Read the model definition and answer for the solid it produces. Units are mm, in the model's axes. Face numbers are marked on the shaded views. A direction names the side the tool comes from. Coordinates: 2 decimals unless noted, no trailing zeros. Write each loop counter-clockwise with the first axis right and the second up, starting at its lowest first coordinate (ties: lowest second). Pieces come first, ordered by that corner, then holes. Notation, with made-up numbers: (42, 62.5) -> (91, 62.5) arc R13 cw to (91, 73.5) -> close; hole circle Ø2 at (42.5, 57.5). An arc over 180 degrees is marked (long way). Return JSON: item names as keys, results as strings.
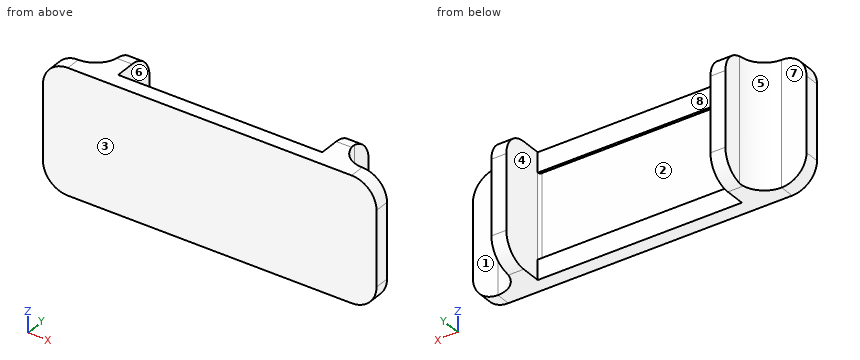
from build123d import *

# Parameters (mm, degrees)
BOSS_EXTRUDE1_DEPTH = 50
FILLET1_R           = 10
FILLET2_R           = 10
SKETCH2_W           = 82
SKETCH2_H           = 34
CUT_EXTRUDE1_DEPTH  = 1
FILLET3_R           = 1


with BuildPart() as part:
    # Sketch1 → Boss-Extrude1 (new body)
    with BuildSketch(Plane.XY):
        Polygon((0, 0), (82, 0), (82, 18), (88, 18), (88, 0), (108, 0), (108, -6), (0, -6), (-6, -6), (-26, -6), (-26, 0), (-6, 0), (-6, 18), (0, 18), align=None)
    extrude(amount=BOSS_EXTRUDE1_DEPTH)

    # Fillet1
    fillet1_edges = [part.edges().sort_by_distance(p)[0] for p in [
        (88, 0, 25),
        (-6, 0, 25),
        (108, -3, 0),
        (108, -3, 50),
        (-26, -3, 0),
        (-26, -3, 50),
    ]]
    fillet(fillet1_edges, radius=FILLET1_R - 0.0001)  # a hair under: the kernel refuses the full size

    # Fillet2
    fillet2_edges = [part.edges().sort_by_distance(p)[0] for p in [
        (85, 18, 50),
        (85, 18, 0),
        (-3, 18, 0),
        (-3, 18, 50),
    ]]
    fillet(fillet2_edges, radius=FILLET2_R)

    # Sketch2 → Cut-Extrude1 (cut)
    with BuildSketch(Plane(origin=(0, 0, 0), x_dir=(1, 0, 0), z_dir=(0, 1, 0))):
        with Locations((41, -25)):
            Rectangle(SKETCH2_W, SKETCH2_H)
    extrude(amount=-CUT_EXTRUDE1_DEPTH, mode=Mode.SUBTRACT)

    # Fillet3
    fillet3_edges = [part.edges().sort_by_distance(p)[0] for p in [
        (82, -1, 25),
        (0, -1, 25),
    ]]
    fillet(fillet3_edges, radius=FILLET3_R)


solid = part.part
1. The part is cut by section B-B (y = 3.5). Determine the outline of the cut face in (x, z), then the cut area to 3 significant figures.
Taken from the geometry:
{"outline": "(-8.4, 0) -> (0, 0) -> (0, 50) -> (-8.4, 50) -> close; (82, 0) -> (90.4, 0) -> (90.4, 50) -> (82, 50) -> close", "area": "840 mm2"}
2. The part is cut by section C-C (z = 21). Determine the outline of the cut face in (x, y).
Taken from the geometry:
{"outline": "(-26, -6) -> (108, -6) -> (108, 0) -> (98, 0) arc R10 cw to (88, 10) -> (88, 18) -> (82, 18) -> (82, 0) arc R1 cw to (81, -1) -> (1, -1) arc R1 cw to (0, 0) -> (0, 18) -> (-6, 18) -> (-6, 10) arc R10 cw to (-16, 0) -> (-26, 0) -> close"}
3. A tool of negligible diameter and unlimited length cuts with its end or side. For the marked faces 1, 2, 3 and 4, from which of +Z, -Z, +X, -X, +Y, -Y can it reach the whole face along a straight path? Write none if from no direction.
Taken from the geometry:
{"face 1": "+Z, -Z, +X, +Y", "face 2": "+Y", "face 3": "+Z, -Z, +X, -X, -Y", "face 4": "+Z, -Z, +Y"}
4. For a pull along X with two mould halves and no side action, classify the marked faces 5, 6, 7 and 8 as +X half, -X half, draft (parallel to the pull), parting line (faces both ways), or undercut.
Taken from the geometry:
{"face 5": "-X half", "face 6": "undercut", "face 7": "draft", "face 8": "undercut"}
5. Consider L1, parallel to X at y = 13.25, z = 38; L2, parallel to Y at x = 2, z = 3.5; L3, parallel to X at y = 6, z = 5.5. Determine where each line is inside the solid, lowest interval first.
Taken from the geometry:
{"L1": "x = -6 to 0, 82 to 88", "L2": "y = -6 to 0", "L3": "x = -6.83 to 0, 82 to 88.83"}
6. Flat-ended cylindrical pins translate along their axes: pin 1 Ø9 at (y, z) = (15.5, 17) entering from -X; pin 2 Ø11 at (x, z) = (-23.5, 29) entering from +Y; pin 3 Ø9 at (y, z) = (12.5, 35) entering from +X. Find the tip coordinate at first contact, or state that the pin passes through.
Taken from the geometry:
{"pin 1": "stops at x = -6", "pin 2": "stops at y = 0", "pin 3": "stops at x = 88.2"}
7. The part is cut by section D-D (y = 13.75). Determine the outline of the cut face in (x, z), then the cut area to 3 significant figures.
Taken from the geometry:
{"outline": "(-6, 1.82) -> (0, 1.82) -> (0, 48.18) -> (-6, 48.18) -> close; (82, 1.82) -> (88, 1.82) -> (88, 48.18) -> (82, 48.18) -> close", "area": "556 mm2"}
8. The part is cut by section A-A (x = 6). Determine the outline of the cut face in (y, z).
Taken from the geometry:
{"outline": "(-6, 0) -> (0, 0) -> (0, 8) -> (-1, 8) -> (-1, 42) -> (0, 42) -> (0, 50) -> (-6, 50) -> close"}
